```python
from build123d import *

# Parameters (mm, degrees)
F0_R     = 32
F0_R_2   = 2.5
F1_DEPTH = 5
F2_R     = 9.75
F3_DEPTH = 5.5
F4_R     = 1.5
F5_DEPTH = 4.501
F6_R     = 2
F7_DEPTH = 10.001


with BuildPart() as f1:
    # F0 (on Right) → F1 (new body, symmetric)
    with BuildSketch(Plane.YZ):
        Circle(F0_R)
        Circle(F0_R_2, mode=Mode.SUBTRACT)
    extrude(amount=F1_DEPTH, both=True)

    # F2 (on face) → F3 (cut)
    with BuildSketch(Plane.YZ.offset(5)):
        Circle(F2_R)
    extrude(amount=-F3_DEPTH, mode=Mode.SUBTRACT)

    # F4 (on face) → F5 (cut, through all)
    with BuildSketch(Plane.YZ.offset(-0.5)):
        with Locations((-4.490128, 4.490128)):
            Circle(F4_R)
        with Locations((-4.490128, -4.490128)):
            Circle(F4_R)
        with Locations((4.490128, -4.490128)):
            Circle(F4_R)
        with Locations((4.490128, 4.490128)):
            Circle(F4_R)
    extrude(amount=-F5_DEPTH, mode=Mode.SUBTRACT)

    # F6 (on face) → F7 (cut, through all)
    with BuildSketch(Plane.YZ.offset(5)):
        with Locations((0, 25)):
            Circle(F6_R)
        with Locations((-17.67767, 17.67767)):
            Circle(F6_R)
        with Locations((-25, 0)):
            Circle(F6_R)
        with Locations((-17.67767, -17.67767)):
            Circle(F6_R)
        with Locations((0, -25)):
            Circle(F6_R)
        with Locations((17.67767, -17.67767)):
            Circle(F6_R)
        with Locations((25, 0)):
            Circle(F6_R)
        with Locations((17.67767, 17.67767)):
            Circle(F6_R)
    extrude(amount=-F7_DEPTH, mode=Mode.SUBTRACT)


solid = f1.part
```
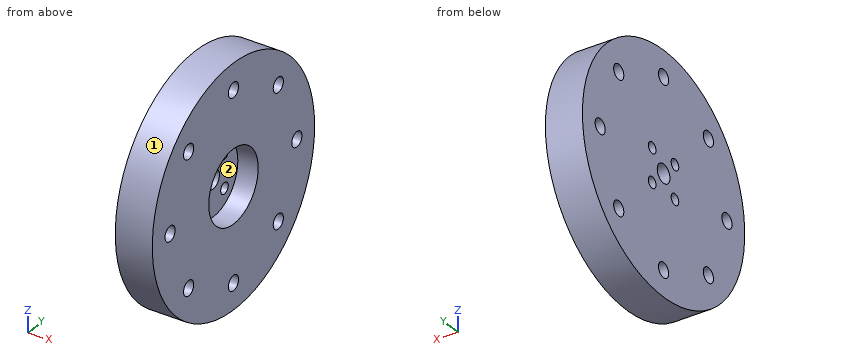
Geometry check sheet. Reference: the model listing, model coordinates, mm. Face numbers are marked on the shaded views. A direction names the side the tool comes from. Coordinates: 2 decimals unless noted, no trailing zeros. Loops run counter-clockwise (first coordinate to the right, second up) from the corner with the lowest first, then second, coordinate; pieces in that order, holes last. Notation, with made-up numbers: (78.5, -30.5) - (90.5, -30.5) arc R20 ccw to (90.5, -23.5) - close; hole circle Ø5 at (46.5, -16). An arc over 180 degrees is marked (long way). One line per item, written item: value. Start each with the question number.
(1) Depth check by flat-ended pin: P1, Ø8, axis at y = 0, z = 0, coming from the +X side; P2, Ø1, axis at x = 3.5, y = -5.5, coming from the +Z side; P3, Ø3, axis at x = -3.5, y = 17.5, coming from the +Z side. Enter the tip coordinate at first touch or a pass-through.
(2) Cross-section at A-A on z = 0. Enter the section's corners in (x, y).
(3) Material ranges on line 1 (Y direction, x = -1, z = -4.5); line 2 (Z direction, x = 0, y = -17); line 3 (Y direction, x = 4, z = 17.5), recorded low to high. Write a range as [from, to].
(4) Tool access check on the marked faces 1 and 2. Record the directions out of +Z, -Z, +X, -X, +Y, -Y that give a thin tool (end or side, any length) a straight path to the whole face; none if there is none.
(5) Cross-section at C-C on y = -25. Enter the section's corners in (x, z).
Results below:
1. P1: stops at x = -0.5
1. P2: stops at z = 31.61
1. P3: stops at z = 27.71
2. outline: (-5, -32) - (5, -32) - (5, -27) - (-5, -27) - close; (-5, -23) - (5, -23) - (5, -9.75) - (-0.5, -9.75) - (-0.5, -2.5) - (-5, -2.5) - close; (-5, 2.5) - (-0.5, 2.5) - (-0.5, 9.75) - (5, 9.75) - (5, 23) - (-5, 23) - close; (-5, 27) - (5, 27) - (5, 32) - (-5, 32) - close
3. line 1: y = [-31.68, -5.99], [-2.99, 2.99], [5.99, 31.68]
3. line 2: z = [-27.11, -19.56], [-15.8, 15.8], [19.56, 27.11]
3. line 3: y = [-26.79, -19.67], [-15.69, 15.69], [19.67, 26.79]
4. face 1: +X, -X
4. face 2: +X
5. outline: (-5, -19.97) - (5, -19.97) - (5, -2) - (-5, -2) - close; (-5, 2) - (5, 2) - (5, 19.97) - (-5, 19.97) - close
